```python
from build123d import *

# Parameters (mm, degrees)
SKETCH1_W           = 647.7
SKETCH1_H           = 344.678
SKETCH1_R           = 9.779
SKETCH1_W_2         = 27.1018
SKETCH1_H_2         = 19.3548
BOSS_EXTRUDE1_DEPTH = 12.7
FILLET1_R           = 10
FILLET2_R           = 10


with BuildPart() as part:
    # Sketch1 → Boss-Extrude1 (new body)
    with BuildSketch(Plane.XY):
        with Locations((25.51036036, -39.985171171)):
            Rectangle(SKETCH1_W, SKETCH1_H)
        with Locations((-244.559967776, -112.969371171)):
            Circle(SKETCH1_R, mode=Mode.SUBTRACT)
        with BuildLine():
            Line((339.86036036, -207.324171171), (338.86036036, -207.324171171))
            ThreePointArc((338.86036036, -207.324171171), (337.092593407, -206.591938124), (336.36036036, -204.824171171))
            Line((336.36036036, -204.824171171), (336.36036036, -199.824171171))
            ThreePointArc((336.36036036, -199.824171171), (337.092593407, -198.056404218), (338.86036036, -197.324171171))
            Line((338.86036036, -197.324171171), (339.86036036, -197.324171171))
            ThreePointArc((339.86036036, -197.324171171), (341.628127313, -198.056404218), (342.36036036, -199.824171171))
            Line((342.36036036, -199.824171171), (342.36036036, -204.824171171))
            ThreePointArc((342.36036036, -204.824171171), (341.628127313, -206.591938124), (339.86036036, -207.324171171))
        make_face(mode=Mode.SUBTRACT)
        with BuildLine():
            Line((-287.83963964, -207.324171171), (-288.83963964, -207.324171171))
            ThreePointArc((-288.83963964, -207.324171171), (-290.607406593, -206.591938124), (-291.33963964, -204.824171171))
            Line((-291.33963964, -204.824171171), (-291.33963964, -199.824171171))
            ThreePointArc((-291.33963964, -199.824171171), (-290.607406593, -198.056404218), (-288.83963964, -197.324171171))
            Line((-288.83963964, -197.324171171), (-287.83963964, -197.324171171))
            ThreePointArc((-287.83963964, -197.324171171), (-286.071872687, -198.056404218), (-285.33963964, -199.824171171))
            Line((-285.33963964, -199.824171171), (-285.33963964, -204.824171171))
            ThreePointArc((-285.33963964, -204.824171171), (-286.071872687, -206.591938124), (-287.83963964, -207.324171171))
        make_face(mode=Mode.SUBTRACT)
        with BuildLine():
            Line((-287.83963964, 117.355828829), (-288.83963964, 117.355828829))
            ThreePointArc((-288.83963964, 117.355828829), (-290.607406593, 118.088061876), (-291.33963964, 119.855828829))
            Line((-291.33963964, 119.855828829), (-291.33963964, 124.855828829))
            ThreePointArc((-291.33963964, 124.855828829), (-290.607406593, 126.623595782), (-288.83963964, 127.355828829))
            Line((-288.83963964, 127.355828829), (-287.83963964, 127.355828829))
            ThreePointArc((-287.83963964, 127.355828829), (-286.071872687, 126.623595782), (-285.33963964, 124.855828829))
            Line((-285.33963964, 124.855828829), (-285.33963964, 119.855828829))
            ThreePointArc((-285.33963964, 119.855828829), (-286.071872687, 118.088061876), (-287.83963964, 117.355828829))
        make_face(mode=Mode.SUBTRACT)
        with BuildLine():
            Line((339.86036036, 117.355828829), (338.86036036, 117.355828829))
            ThreePointArc((338.86036036, 117.355828829), (337.092593407, 118.088061876), (336.36036036, 119.855828829))
            Line((336.36036036, 119.855828829), (336.36036036, 124.855828829))
            ThreePointArc((336.36036036, 124.855828829), (337.092593407, 126.623595782), (338.86036036, 127.355828829))
            Line((338.86036036, 127.355828829), (339.86036036, 127.355828829))
            ThreePointArc((339.86036036, 127.355828829), (341.628127313, 126.623595782), (342.36036036, 124.855828829))
            Line((342.36036036, 124.855828829), (342.36036036, 119.855828829))
            ThreePointArc((342.36036036, 119.855828829), (341.628127313, 118.088061876), (339.86036036, 117.355828829))
        make_face(mode=Mode.SUBTRACT)
        with Locations((-244.78873964, -162.646771171)):
            Rectangle(SKETCH1_W_2, SKETCH1_H_2, mode=Mode.SUBTRACT)
    extrude(amount=BOSS_EXTRUDE1_DEPTH)

    # Fillet1
    fillet1_edges = [part.edges().sort_by_distance(p)[0] for p in [
        (-298.33963964, 132.353828829, 6.35),
        (349.36036036, 132.353828829, 6.35),
        (349.36036036, -212.324171171, 6.35),
    ]]
    fillet(fillet1_edges, radius=FILLET1_R)

    # Fillet2
    fillet2_edges = [part.edges().sort_by_distance(p)[0] for p in [
        (-298.33963964, -212.324171171, 6.35),
    ]]
    fillet(fillet2_edges, radius=FILLET2_R)


solid = part.part
```
Here's how the part is built. I have some questions about the finished solid (model axes, mm). A direction names the side the tool comes from. Give positions to 0.01 mm unless a question says otherwise; leave off trailing zeros. Return JSON: item names as keys, results as strings.
Item 1: I'm going to push a flat-ended pin straight in: pin 1 Ø11.5 at (x, y) = (-244.56, -112.97) entering from -Z. Where does the tip first touch, or does it pass through?
A:
{"pin 1": "passes through"}
Item 2: Please list where these lines run through material, in increasing order: line 1 (X direction, y = -171.5, z = 3.5); line 2 (Y direction, x = -250.5, z = 8.75).
A:
{"line 1": "x = -298.34 to -258.34, -231.24 to 349.36", "line 2": "y = -212.32 to -172.32, -152.97 to -120.74, -105.2 to 132.35"}
Item 3: On a 3-axis mill with a long thin cutter (end or side, diameter ignored), from which of +Z, -Z, +X, -X, +Y, -Y can I reach the whole of each face in a straight line? I mean faces 1 (the flat face through (-258.34, -163, 6)), 2 (the flat face through (21, -212.324, 6)). Say none if no direction works.
A:
{"face 1": "+Z, -Z", "face 2": "+Z, -Z, +X, -X, -Y"}
Item 4: Thinking about a two-plate mould opening in X: for faces 3 (the flat face through (-298.34, -42, 6)), 4 (the flat face through (-245, -152.969, 6)), 5 (the flat face through (21, 132.354, 6)), 6 (the flat face through (349.36, -42, 6)), which applies, released by +X, released by -X, zero draft, split by the parting line, or undercut?
A:
{"face 3": "released by -X", "face 4": "undercut", "face 5": "zero draft", "face 6": "released by +X"}
